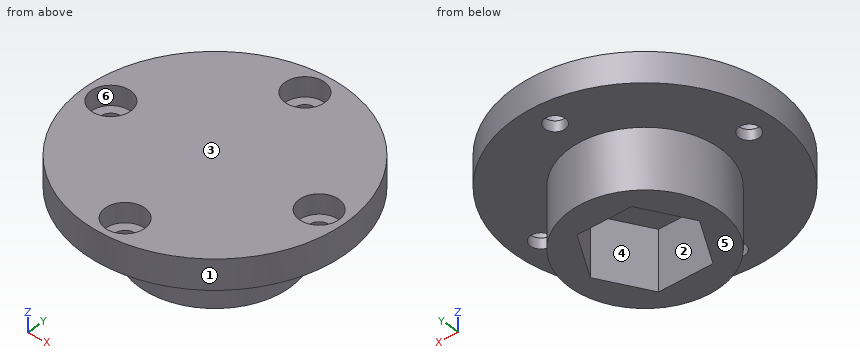
```python
from build123d import *

# Parameters (mm, degrees)
SKETCH1_R           = 10
BOSS_EXTRUDE1_DEPTH = 8
SKETCH2_R           = 17.5
BOSS_EXTRUDE2_DEPTH = 4
CUT_EXTRUDE1_REACH  = 28.01
SKETCH3_R           = 1.375
CIRPATTERN1_COUNT   = 4
SKETCH4_R           = 2.65
CUT_EXTRUDE2_DEPTH  = 2.6
CIRPATTERN2_COUNT   = 4


with BuildPart() as part:
    # Sketch1 → Boss-Extrude1 (new body)
    with BuildSketch(Plane.XY):
        Circle(SKETCH1_R)
        Polygon((7.332348419, 0), (3.666174209, 6.35), (-3.666174209, 6.35), (-7.332348419, 0), (-3.666174209, -6.35), (3.666174209, -6.35), align=None, mode=Mode.SUBTRACT)
    extrude(amount=BOSS_EXTRUDE1_DEPTH)

    # Sketch2 → Boss-Extrude2 (add)
    with BuildSketch(Plane.XY.offset(8)):
        Circle(SKETCH2_R)
    extrude(amount=BOSS_EXTRUDE2_DEPTH)

    # Sketch3 → Cut-Extrude1 (cut, up to next)
    with BuildSketch(Plane(origin=(0, 0, 8), x_dir=(-1, 0, 0), z_dir=(0, 0, -1)), mode=Mode.PRIVATE) as cut_extrude1_sk1:
        with Locations((0, 14)):
            Circle(SKETCH3_R)
    cut_extrude1_tool1 = extrude(cut_extrude1_sk1.sketch, amount=-CUT_EXTRUDE1_REACH, mode=Mode.PRIVATE) & part.part
    cut_extrude1 = cut_extrude1_tool1.solids().sort_by_distance((0, 14, 8))[0]
    add(cut_extrude1, mode=Mode.SUBTRACT)

    # CirPattern1: Cut-Extrude1 ×4 about axis
    cirpattern1_axis = Axis((0, 0, 0), (0, 0, 1))
    for i in range(1, CIRPATTERN1_COUNT):
        add(cut_extrude1.rotate(cirpattern1_axis, i * 360 / CIRPATTERN1_COUNT), mode=Mode.SUBTRACT)

    # Sketch4 → Cut-Extrude2 (cut)
    with BuildSketch(Plane.XY.offset(12)):
        with Locations((0, 14)):
            Circle(SKETCH4_R)
    cut_extrude2 = extrude(amount=-CUT_EXTRUDE2_DEPTH, mode=Mode.SUBTRACT)

    # CirPattern2: Cut-Extrude2 ×4 about axis
    cirpattern2_axis = Axis((0, 0, 0), (0, 0, 1))
    for i in range(1, CIRPATTERN2_COUNT):
        add(cut_extrude2.rotate(cirpattern2_axis, i * 360 / CIRPATTERN2_COUNT), mode=Mode.SUBTRACT)


solid = part.part
```
Input: part model. Units: mm. Frame: model coordinates. Face numbers are marked on the shaded views. A direction names the side the tool comes from. Coordinates: 2 decimals unless noted, no trailing zeros. Loops run counter-clockwise (first coordinate to the right, second up) from the corner with the lowest first, then second, coordinate; pieces in that order, holes last.
Q1. Section A-A, the plane x = 0. Return the cut outline in (y, z) (3 decimals).
Results are:
outline: (-17.5, 8) - (-15.375, 8) - (-15.375, 9.4) - (-16.65, 9.4) - (-16.65, 12) - (-17.5, 12) - close; (-12.625, 8) - (-10, 8) - (-10, 0) - (-6.35, 0) - (-6.35, 8) - (6.35, 8) - (6.35, 0) - (10, 0) - (10, 8) - (12.625, 8) - (12.625, 9.4) - (11.35, 9.4) - (11.35, 12) - (-11.35, 12) - (-11.35, 9.4) - (-12.625, 9.4) - close; (15.375, 8) - (17.5, 8) - (17.5, 12) - (16.65, 12) - (16.65, 9.4) - (15.375, 9.4) - close
Q2. Line query: line 1 along Y through (x, z) = (0, 8.65) (3 decimals); line 2 along Y through (x, z) = (0, 10.65); line 3 along Z through (x, y) = (-3.5, 3). Output: solid intervals per line, ascending.
Results are:
line 1: y = -17.5 to -15.375, -12.625 to 12.625, 15.375 to 17.5
line 2: y = -17.5 to -16.65, -11.35 to 11.35, 16.65 to 17.5
line 3: z = 8 to 12
Q3. Mould query, pull axis Y, two halves, no side actions, for the marked faces 1, 2 and 3. Classes: +Y half, -Y half, draft (parallel to the pull), parting line (faces both ways), or undercut.
Results are:
face 1: parting line
face 2: undercut
face 3: draft
Q4. Section B-B, the plane x = 14. Return the cut outline in (y, z) (3 decimals).
Results are:
outline: (-10.5, 8) - (-1.375, 8) - (-1.375, 9.4) - (-2.65, 9.4) - (-2.65, 12) - (-10.5, 12) - close; (1.375, 8) - (10.5, 8) - (10.5, 12) - (2.65, 12) - (2.65, 9.4) - (1.375, 9.4) - close
Q5. Contact query for flat-ended pins moving along their axis: pin 1 (4.5 mm diameter, centred on x = 0, y = -14, fed in from -Z); pin 2 (1.6 mm diameter, centred on x = -0.5, y = 13.5, fed in from +Z); pin 3 (1 mm diameter, centred on x = 6, z = 3, fed in from -Y). Output: stop coordinate, or through.
Results are:
pin 1: stops at z = 8
pin 2: stops at z = 9.4
pin 3: stops at y = -8.35
Q6. Set-up query: the marked faces 4, 5 and 6. Return all of +Z, -Z, +X, -X, +Y, -Y with unobstructed straight access to the full face (end or side cutting, diameter ignored); none if empty.
Results are:
face 4: -Z
face 5: -Z, +X, -X, +Y, -Y
face 6: +Z
Q7. Section D-D, the plane y = -2. Return the cut outline in (x, z).
Results are:
outline: (-17.39, 8) - (-9.8, 8) - (-9.8, 0) - (-6.18, 0) - (-6.18, 8) - (6.18, 8) - (6.18, 0) - (9.8, 0) - (9.8, 8) - (17.39, 8) - (17.39, 12) - (15.74, 12) - (15.74, 9.4) - (12.26, 9.4) - (12.26, 12) - (-12.26, 12) - (-12.26, 9.4) - (-15.74, 9.4) - (-15.74, 12) - (-17.39, 12) - close
